Can you work these out from the model? Positions are in its coordinate system, mm. A direction names the side the tool comes from. Round coordinates to 2 decimals unless told otherwise and drop trailing zeros. Loops run counter-clockwise (first coordinate to the right, second up) from the corner with the lowest first, then second, coordinate; pieces in that order, holes last. Notation, with made-up numbers: (-29, 60.5) -> (3, 60.5) arc R23 ccw to (3, 94.5) -> close; hole circle Ø11 at (3.25, 30.5). An arc over 180 degrees is marked (long way). Answer as a JSON object with one key per item and string values.
```python
from build123d import *

# Parameters (mm, degrees)
SKETCH_1_R          = 10.25
SKETCH_1_R_2        = 1.5
EXTRUDE_1_DEPTH     = 2
SKETCH_2_R          = 4
EXTRUDE_2_DEPTH     = 3
SKETCH_3_R          = 2.5
CUT_EXTRUDE_1_DEPTH = 3
FILLET_1_R          = 0.5
FILLET_2_R          = 0.5
FILLET_3_R          = 0.5


with BuildPart() as part:
    # 草图1 → 凸台-拉伸1 (new body)
    with BuildSketch(Plane.XY):
        Circle(SKETCH_1_R)
        Circle(SKETCH_1_R_2, mode=Mode.SUBTRACT)
        with Locations((-7.35, 0)):
            Circle(SKETCH_1_R_2, mode=Mode.SUBTRACT)
        with Locations((7.35, 0)):
            Circle(SKETCH_1_R_2, mode=Mode.SUBTRACT)
        with Locations((0, 7.35)):
            Circle(SKETCH_1_R_2, mode=Mode.SUBTRACT)
        with Locations((0, -7.35)):
            Circle(SKETCH_1_R_2, mode=Mode.SUBTRACT)
    extrude(amount=EXTRUDE_1_DEPTH)

    # 草图2 → 凸台-拉伸2 (add)
    with BuildSketch(Plane.XY.offset(2)):
        Circle(SKETCH_2_R)
    extrude(amount=EXTRUDE_2_DEPTH)

    # 草图3 → 切除-拉伸1 (cut)
    with BuildSketch(Plane.XY.offset(5)):
        Circle(SKETCH_3_R)
    extrude(amount=-CUT_EXTRUDE_1_DEPTH, mode=Mode.SUBTRACT)

    # 圆角1
    fillet_1_edges = [part.edges().sort_by_distance(p)[0] for p in [
        (-10.25, 0, 2),
    ]]
    fillet(fillet_1_edges, radius=FILLET_1_R)

    # 圆角2
    fillet_2_edges = [part.edges().sort_by_distance(p)[0] for p in [
        (-10.25, 0, 0),
    ]]
    fillet(fillet_2_edges, radius=FILLET_2_R)

    # 圆角3
    fillet_3_edges = [part.edges().sort_by_distance(p)[0] for p in [
        (-4, 0, 5),
    ]]
    fillet(fillet_3_edges, radius=FILLET_3_R)


solid = part.part
```
Q1. I want a section at A-A, the plane y = 0. Give the number of separate pieces and of enclosed holes in the cut face, then the cut area to 3 significant figures.
Determined:
{"separate pieces": "4", "enclosed holes": "0", "area": "31.7 mm²"}
Q2. I want a section at C-C, the plane z = 3.1. Write out the boundary of the cut face in (x, y), then the cut area to 3 significant figures.
Determined:
{"outline": "circle Ø8 at (0, 0); hole circle Ø5 at (0, 0)", "area": "30.6 mm²"}
Q3. I'm going to push flat-ended pins straight in: pin 1 (5 mm diameter, centred on x = 7.35, y = 0, fed in from +Z); pin 2 (2 mm diameter, centred on x = -8, y = 7.5, fed in from -Z); pin 3 (3 mm diameter, centred on y = -2, z = 0.5, fed in from +X). Where does each tip first touch, or does it pass through?
Determined:
{"pin 1": "z = 2", "pin 2": "z = 0.05", "pin 3": "x = 10.24"}
Q4. On a 3-axis mill with a long thin cutter (end or side, diameter ignored), from which of +Z, -Z, +X, -X, +Y, -Y can I reach the whole of each face in a straight line? I mean faces 1 (the flat face through (4.2, 0.1, 2)), 2 (the cylindrical face through (8.736, -0.575, 0.986)). Say none if no direction works.
Determined:
{"face 1": "+Z", "face 2": "+Z, -Z"}
Q5. If I drill on L1, parallel to Y at x = 0, z = 1.3; L2, parallel to Y at x = 0, z = 2.85; L3, parallel to Y at x = 1, z = 0.3, over which ranges is the centre line in solid material (lowest first)? Write a range as [from, to].
Determined:
{"L1": "[-10.25, -8.85], [-5.85, -1.5], [1.5, 5.85], [8.85, 10.25]", "L2": "[-4, -2.5], [2.5, 4]", "L3": "[-10.16, -8.47], [-6.23, -1.12], [1.12, 6.23], [8.47, 10.16]"}
Q6. We'd pull the mould along X, two halves only. Please class faces 3 (the flat face through (0, -2, 2)), 4 (the flat face through (2, -2, 5)), 5 (the cylindrical face through (-2.222, -10.006, 0.993)): pulls with the +X half, pulls with the -X half, needs draft (parallel to the pull), parting line crosses it, or undercut.
Determined:
{"face 3": "undercut", "face 4": "needs draft", "face 5": "parting line crosses it"}
